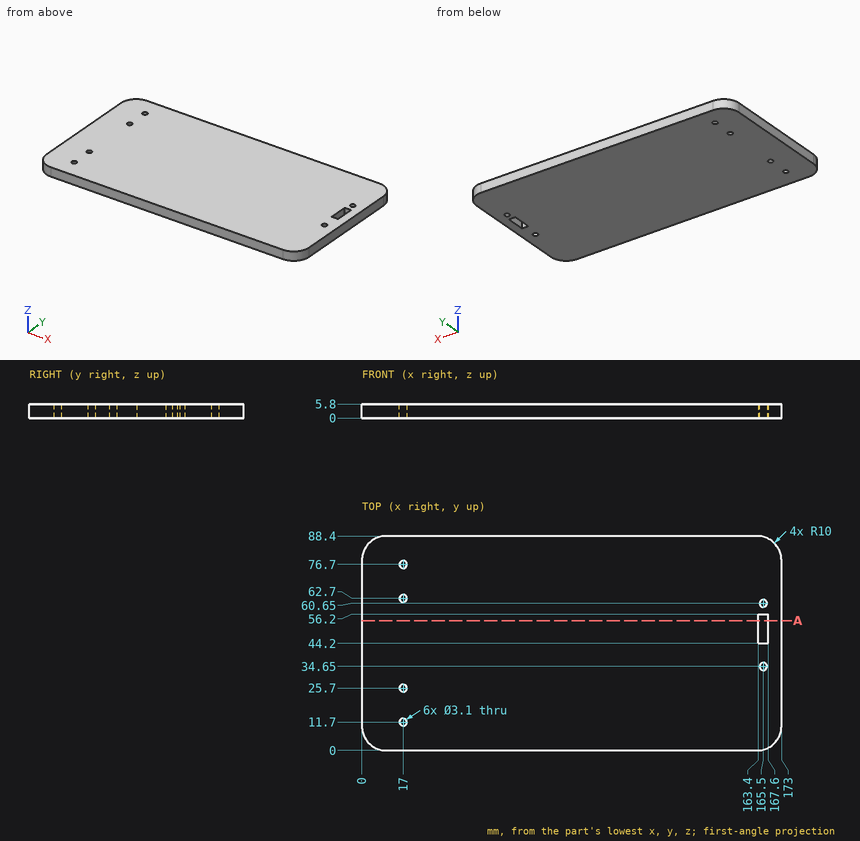
The figure shows three views and two pictorial views of one solid part (mm, origin at its lowest corner). Answer the questions. Coordinates: 2 decimals unless noted, no trailing zeros. Loops run counter-clockwise (first coordinate to the right, second up) from the corner with the lowest first, then second, coordinate; pieces in that order, holes last. Notation, with made-up numbers: (-34, 40.5) -> (5, 40.5) arc R32 cw to (5, 71.5) -> close; hole circle Ø6 at (47, 30.25). An arc over 180 degrees is marked (long way). Use one line per item in the form item = value. Start each with the question number.
Item 1: The part is cut by section A-A on y = 53.5. Determine the outline of the cut face in (x, z).
Item 2: Flat-ended cylindrical pins translate along their axes: pin 1 Ø2.5 at (x, y) = (17, 25.7) entering from -Z; pin 2 Ø2 at (x, z) = (165, 3) entering from +Y. Find the tip coordinate at first contact, or state that the pin passes through.
Item 3: Consider L1, parallel to Y at x = 17, z = 4.1; L2, parallel to X at y = 49.5, z = 1.4; L3, parallel to Y at x = 165.5, z = 1.75. Determine where each line is inside the solid, lowest interval first. Write a range as [from, to].
Answer key:
q1.outline = (0, 0) -> (163.4, 0) -> (163.4, 5.8) -> (0, 5.8) -> close; (167.6, 0) -> (173, 0) -> (173, 5.8) -> (167.6, 5.8) -> close
q2.pin_1 = through
q2.pin_2 = 88.35
q3.L1 = [0, 10.15], [13.25, 24.15], [27.25, 61.15], [64.25, 75.15], [78.25, 88.4]
q3.L2 = [0, 163.4], [167.6, 173]
q3.L3 = [0.32, 33.1], [36.2, 44.2], [56.2, 59.1], [62.2, 88.08]
